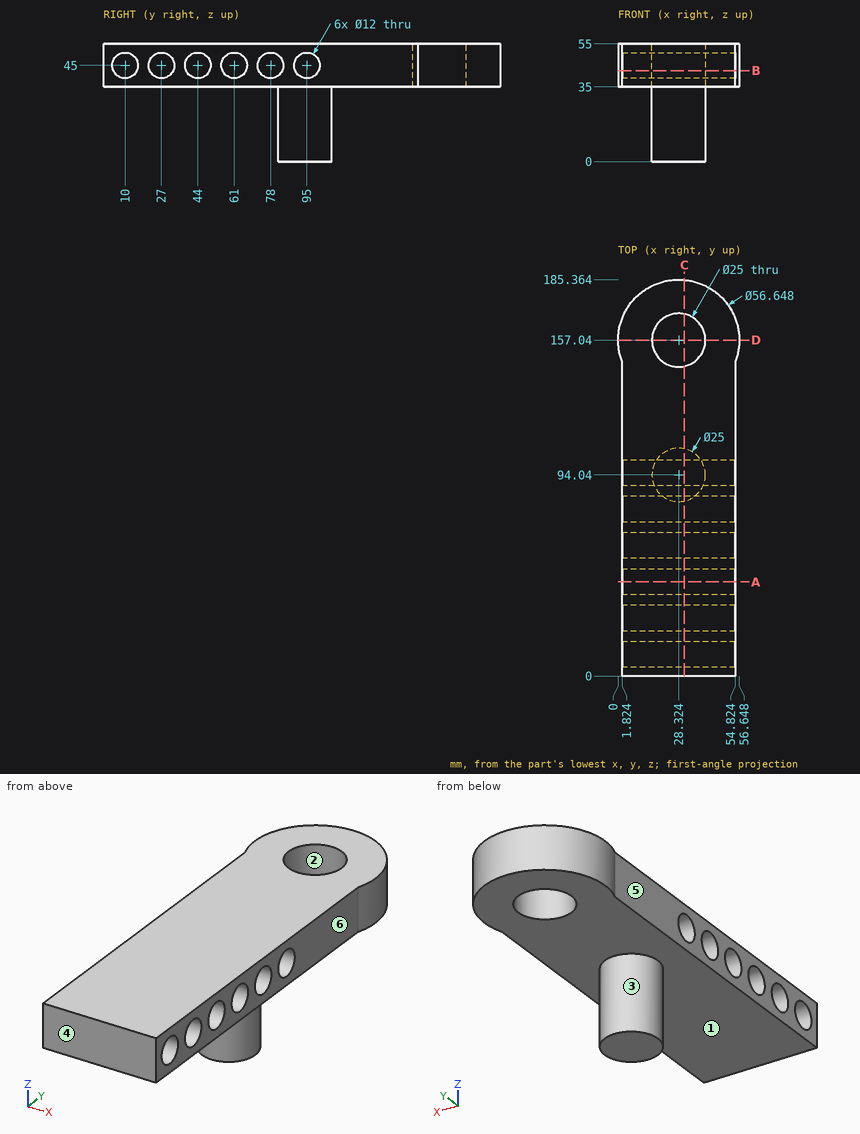
Geometry check sheet. Reference: drawing and pictorial views, mm from the part's lowest x, y, z. A direction names the side the tool comes from. Give positions to 0.01 mm unless a question says otherwise; leave off trailing zeros. Order: outer loops, then holes, each group sorted by start corner. A loop starts at its lowest first (then second) coordinate and runs counter-clockwise, first axis right, second up. Notation, with made-up numbers: (-10.75, -22) - (13.25, -22) arc R26 ccw to (13.25, 8) - close; hole circle Ø6 at (9.5, -28). An arc over 180 degrees is marked (long way). Answer as CSV lines item,"result". Start each with the question number.
Item 1: Section check D-D, the plane y = 157.04. Record the boundary of the cut face in (x, z).
Item 2: Gauge pin test, flat ends, axial feed: pin 1 (22 mm diameter, centred on y = 40, z = 41.5, fed in from -X); pin 2 (10 mm diameter, centred on x = 44, z = 25.5, fed in from -Y); pin 3 (2 mm diameter, centred on x = 18.5, z = 18, fed in from +Y). Record the tip position at first contact, or that the pin passes through.
Item 3: Material ranges on L1, parallel to X at y = 46, z = 51.5; L2, parallel to Z at x = 51.5, y = 102; L3, parallel to X at y = 167, z = 41, recorded low to high.
Item 4: Section check C-C, the plane x = 31. Record the boundary of the cut face in (y, z), plus the area to 3 significant figures.
Item 5: Section check A-A, the plane y = 44. Record the boundary of the cut face in (x, z), plus the area to 3 significant figures.
Item 6: Mould release check, pull along X, two halves, no side actions. Record for the marked faces 1, 2 and 3: released by +X, released by -X, zero draft, split by the parting line, or undercut.
Item 7: Access from +Z, -Z, +X, -X, +Y, -Y to the whole of each face (thin tool, end or side, straight path). Record for the marked faces 4, 5 and 6.
Item 8: Section check B-B, the plane z = 42.5. State how many separate pieces and enclosed holes the cut face has, plus the area to 3 significant figures.
Filled in:
1,outline,"(0, 35) - (15.82, 35) - (15.82, 55) - (0, 55) - close; (40.82, 35) - (56.65, 35) - (56.65, 55) - (40.82, 55) - close"
2,pin 1,"x = 1.82"
2,pin 2,"y = 87.54"
2,pin 3,"y = 102.89"
3,L1,"1.82 to 54.82"
3,L2,"35 to 55"
3,L3,"1.81 to 20.77, 35.88 to 54.84"
4,outline,"(0, 35) - (81.83, 35) - (81.83, 0) - (106.25, 0) - (106.25, 35) - (144.83, 35) - (144.83, 55) - (0, 55) - close; (169.25, 35) - (185.24, 35) - (185.24, 55) - (169.25, 55) - close; hole circle Ø12 at (10, 45); hole circle Ø12 at (27, 45); hole circle Ø12 at (44, 45); hole circle Ø12 at (61, 45); hole circle Ø12 at (78, 45); hole circle Ø12 at (95, 45)"
4,area,"3,390 mm^2"
5,outline,"(1.82, 35) - (54.82, 35) - (54.82, 39) - (1.82, 39) - close; (1.82, 51) - (54.82, 51) - (54.82, 55) - (1.82, 55) - close"
5,area,"424 mm^2"
6,face 1,"zero draft"
6,face 2,"undercut"
6,face 3,"split by the parting line"
7,face 4,"+Z, -Z, +X, -X, -Y"
7,face 5,"+Z, -Z, -X, -Y"
7,face 6,"+Z, -Z, +X, -Y"
8,separate pieces,"7"
8,enclosed holes,"1"
8,area,"5,650 mm^2"
